```python
from build123d import *

# Parameters (mm, degrees)
BOSS_EXTRUDE1_DEPTH = 3.175


with BuildPart() as part:
    # Sketch1 → Boss-Extrude1 (new body)
    with BuildSketch(Plane.XY):
        with BuildLine():
            Line((0, 82.55), (0, 53.594))
            Line((0, 53.594), (3.683, 53.594))
            Line((3.683, 53.594), (3.683, 55.245))
            Line((3.683, 55.245), (6.477, 55.245))
            Line((6.477, 55.245), (6.477, 48.895))
            Line((6.477, 48.895), (3.683, 48.895))
            Line((3.683, 48.895), (3.683, 50.546))
            Line((3.683, 50.546), (0, 50.546))
            Line((0, 50.546), (0, 21.59))
            Line((0, 21.59), (-3.175, 21.59))
            Line((-3.175, 21.59), (-3.175, 2.54))
            Line((-3.175, 2.54), (0, 2.54))
            ThreePointArc((0, 2.54), (0.743948776, 0.743948776), (2.54, 0))
            Line((2.54, 0), (82.55, 0))
            add(Edge.make_bspline(
                [(0, 104.14), (20.815651588, 104.14), (82.55, 29.560059324), (82.55, 0)],
                knots=[0, 0, 0, 0, 1, 1, 1, 1], degree=3))
            Line((0, 104.14), (0, 101.6))
            Line((0, 101.6), (-3.175, 101.6))
            Line((-3.175, 101.6), (-3.175, 82.55))
            Line((-3.175, 82.55), (0, 82.55))
        make_face()
        with BuildLine():
            Line((19.05, 72.527700628), (19.05, 19.05))
            Line((19.05, 19.05), (58.0732756, 19.05))
            add(Edge.make_bspline(
                [(19.05, 72.527700628), (24.979605929, 68.637560894), (52.981970502, 35.459305466), (58.0732756, 19.05)],
                knots=[0, 0, 0, 0, 1, 1, 1, 1], degree=3))
        make_face(mode=Mode.SUBTRACT)
    extrude(amount=BOSS_EXTRUDE1_DEPTH)


solid = part.part
```
Could you check a few things on this model? Use its own coordinates, in mm. A direction names the side the tool comes from. Give positions to 0.01 mm unless a question says otherwise; leave off trailing zeros. Use one line per item in the form item = value.
1. I'm going to push flat-ended pins straight in: pin 1 Ø1 at (x, z) = (30, 1.5) entering from +Y; pin 2 Ø1 at (x, z) = (1.5, 2) entering from -Y; pin 3 Ø1 at (y, z) = (52.5, 1) entering from -X. Where does each tip first touch, or does it pass through?
Response values:
pin_1 = 84.85
pin_2 = 0.06
pin_3 = 6.48
2. On a 3-axis mill with a long thin cutter (end or side, diameter ignored), from which of +Z, -Z, +X, -X, +Y, -Y can I reach the whole of each face in a straight line? I mean faces 1 (the face through (5, 55.245, 2)), 2 (the face through (-2, 82.55, 2)), 3 (the face through (-2, 2.54, 2)), 4 (the face through (0, 103, 2)). Say none if no direction works.
Response values:
face_1 = +Z, -Z
face_2 = +Z, -Z, -X
face_3 = +Z, -Z, -X, -Y
face_4 = +Z, -Z, -X, +Y
3. Thinking about a two-plate mould opening in X: for faces 5 (the face through (19.05, 46, 2)), 6 (the face through (0.724, 0.764, 1.565)), 7 (the face through (2, 53.594, 2)), which applies, released by +X, released by -X, zero draft, split by the parting line, or undercut?
Response values:
face_5 = undercut
face_6 = released by -X
face_7 = zero draft
4. I need wall thicknesses on probe 1 along X at (y, z) = (21.5, 1.55) (3 decimals); probe 2 along Y at (x, z) = (56.5, 1.3); probe 3 along Y at (x, z) = (42.5, 0.3). Which ranges of each line are inside material? Lowest first, please.
Response values:
probe_1 = -3.175 to 19.05, 57.196 to 76.288
probe_2 = 0 to 19.05, 23.14 to 53.55
probe_3 = 0 to 19.05, 45.69 to 71.01
